Here's the drawing with two shaded views (mm, measured from the low corner). I have some questions. A direction names the side the tool comes from. Coordinates: 2 decimals unless noted, no trailing zeros. Order: outer loops, then holes, each group sorted by start corner. A loop starts at its lowest first (then second) coordinate and runs counter-clockwise, first axis right, second up. Notation, with made-up numbers: (62, 89.25) -> (101, 89.25) arc R17 cw to (101, 118.25) -> close; hole circle Ø11 at (51, 22). An arc over 180 degrees is marked (long way). One line per item, written item: value. Start each with the question number.
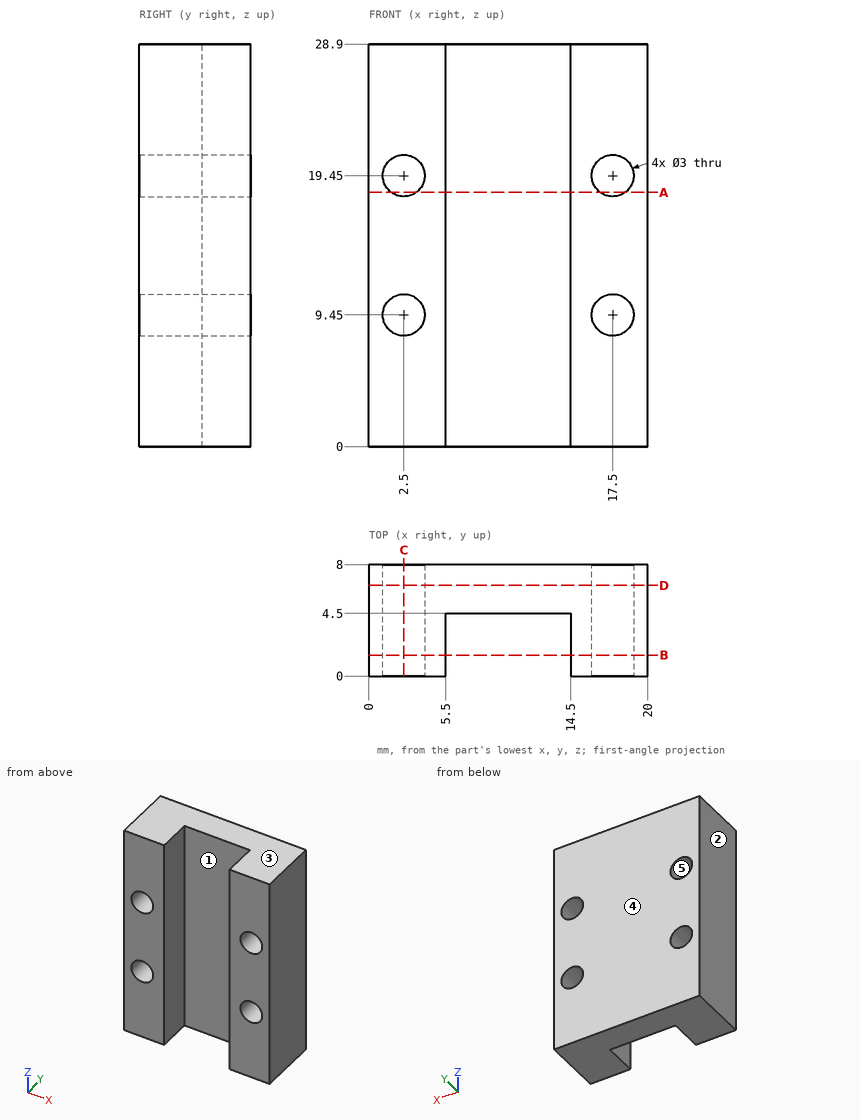
Q1. Imagine slicing it at D-D (y = 6.5). Write out the boundary of the cut face in (x, z), plus the area to 3 significant figures.
Q2. For the marked faces 1 and 2, which set-ups out of +Z, -Z, +X, -X, +Y, -Y let a thin tool reach every point of the face, with its end or its side?
Q3. Imagine slicing it at B-B (y = 1.5). Write out the boundary of the cut face in (x, z), plus the area to 3 significant figures.
Q4. Imagine slicing it at A-A (z = 18.25). Write out the boundary of the cut face in (x, y), plus the area to 3 significant figures.
Q5. Imagine slicing it at C-C (x = 2.5). Write out the boundary of the cut face in (y, z), plus the area to 3 significant figures.
Q6. I need wall thicknesses on line 1 (Z direction, x = 2.5, y = 2.75); line 2 (X direction, y = 0.5, z = 22); line 3 (X direction, y = 5.25, z = 9.45). Which ranges of each line are inside material? Lowest first, please.
Q7. For P1, Ø2.5, axis at x = 2.5, z = 9.45, coming from the +Y side; P2, Ø5, axis at x = 10, z = 5.5, coming from the -Y side, each with a flat end and sliding along its axis, tell me the tip position at first contact or that it passes through.
Q8. If we mould it in two halves opening along Z, with no side actions, what happens to the marked faces 3, 4 and 5? For each: +Z half, -Z half, draft (parallel to the pull), parting line (faces both ways), or undercut.
Completed:
1. outline: (0, 0) -> (20, 0) -> (20, 28.9) -> (0, 28.9) -> close; hole circle Ø3 at (2.5, 9.45); hole circle Ø3 at (2.5, 19.45); hole circle Ø3 at (17.5, 9.45); hole circle Ø3 at (17.5, 19.45)
1. area: 550 mm2
2. face 1: +Z, -Z, -Y
2. face 2: +Z, -Z, -X, +Y, -Y
3. outline: (0, 0) -> (5.5, 0) -> (5.5, 28.9) -> (0, 28.9) -> close; (14.5, 0) -> (20, 0) -> (20, 28.9) -> (14.5, 28.9) -> close; hole circle Ø3 at (2.5, 9.45); hole circle Ø3 at (2.5, 19.45); hole circle Ø3 at (17.5, 9.45); hole circle Ø3 at (17.5, 19.45)
3. area: 290 mm2
4. outline: (0, 0) -> (1.6, 0) -> (1.6, 8) -> (0, 8) -> close; (3.4, 0) -> (5.5, 0) -> (5.5, 4.5) -> (14.5, 4.5) -> (14.5, 0) -> (16.6, 0) -> (16.6, 8) -> (3.4, 8) -> close; (18.4, 0) -> (20, 0) -> (20, 8) -> (18.4, 8) -> close
4. area: 90.7 mm2
5. outline: (0, 0) -> (8, 0) -> (8, 7.95) -> (0, 7.95) -> close; (0, 10.95) -> (8, 10.95) -> (8, 17.95) -> (0, 17.95) -> close; (0, 20.95) -> (8, 20.95) -> (8, 28.9) -> (0, 28.9) -> close
5. area: 183 mm2
6. line 1: z = 0 to 7.95, 10.95 to 17.95, 20.95 to 28.9
6. line 2: x = 0 to 5.5, 14.5 to 20
6. line 3: x = 0 to 1, 4 to 16, 19 to 20
7. P1: passes through
7. P2: stops at y = 4.5
8. face 3: +Z half
8. face 4: draft
8. face 5: undercut
